Geometry: final body of the model. Coordinates: model frame, mm. Face numbers are marked on the shaded views. A direction names the side the tool comes from. Give positions to 0.01 mm unless a question says otherwise; leave off trailing zeros. Loops run counter-clockwise (first coordinate to the right, second up) from the corner with the lowest first, then second, coordinate; pieces in that order, holes last. Notation, with made-up numbers: (-38.5, 67.5) -> (-2.5, 67.5) arc R23 cw to (-2.5, 82.5) -> close; hole circle Ø1 at (52, 73.25). An arc over 180 degrees is marked (long way). One line per item, written item: value. Start each with the question number.
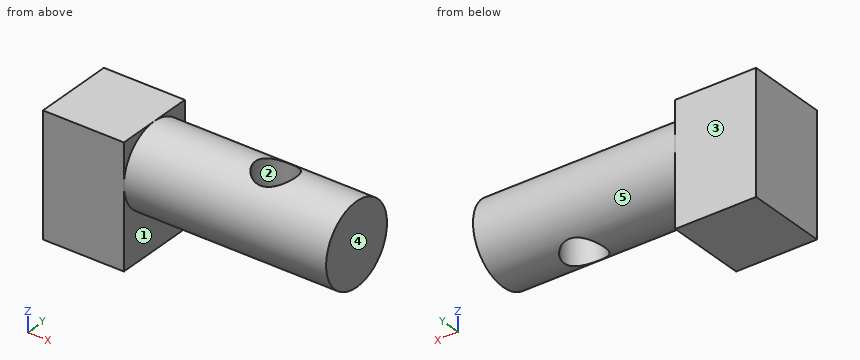
from build123d import *

# Parameters (mm, degrees)
F0_W     = 20
F0_H     = 30
F1_DEPTH = 20
F2_R     = 10
F3_DEPTH = 50
F4_R     = 5
F5_DEPTH = 30.001


with BuildPart() as f1:
    # F0 (on Front) → F1 (new body)
    with BuildSketch(Plane.XZ):
        Rectangle(F0_W, F0_H)
    extrude(amount=F1_DEPTH)

    # F2 (on face) → F3 (join)
    with BuildSketch(Plane.YZ.offset(10)):
        with Locations((-10, 5)):
            Circle(F2_R)
    extrude(amount=F3_DEPTH)

    # F4 (on face) → F5 (cut, through all)
    with BuildSketch(Plane(origin=(0, 0, -15), x_dir=(1, 0, 0), z_dir=(0, 0, -1))):
        with Locations((40, 10)):
            Circle(F4_R)
    extrude(amount=-F5_DEPTH, mode=Mode.SUBTRACT)


solid = f1.part
Item 1: Ray query, line 1 along X through (y, z) = (-10, 1.5); line 2 along Y through (x, z) = (40, 6); line 3 along X through (y, z) = (-14, -5). Return the intervals inside material, ascending. Write a range as [from, to].
Item 2: Mould query, pull axis Y, two halves, no side actions, for the marked faces 1, 2 and 3. Classes: pulls with the +Y half, pulls with the -Y half, needs draft (parallel to the pull), parting line crosses it, or undercut.
Item 3: Access query for the marked faces 4 and 5. Directions: +Z, -Z, +X, -X, +Y, -Y. A direction counts if a zero-diameter tool reaches every point of the face in a straight line with its end or side. Return the directions, or none.
Item 4: Section A-A, the plane z = 3.5. Output: boundary loops of the cut face in (x, y).
Item 5: Section B-B, the plane y = -13.25. Output: boundary loops of the cut face in (x, z), then the cut area to 3 significant figures.
Item 6: Pin query (flat end, axial travel): pin 1 (9 mm diameter, centred on x = 40, y = -10, fed in from +Z); pin 2 (12 mm diameter, centred on x = 47, y = -5.5, fed in from -Z); pin 3 (3 mm diameter, centred on x = 20.5, y = -17, fed in from +Z); pin 4 (1.5 mm diameter, centred on x = 37, z = 5.5, fed in from -Y). Return the tip coordinate at first contact, or that it passes through.
Item 7: Section D-D, the plane x = 27.5. Output: boundary loops of the cut face in (y, z), then the cut area to 3 significant figures.
Item 8: Section C-C, the plane y = -16.25. Output: boundary loops of the cut face in (x, z), then the cut area to 3 significant figures.
Geometry check:
1. line 1: x = [-10, 35], [45, 60]
1. line 2: y = [-19.95, -15], [-5, -0.05]
1. line 3: x = [-10, 10]
2. face 1: needs draft
2. face 2: undercut
2. face 3: pulls with the +Y half
3. face 4: +Z, -Z, +X, +Y, -Y
3. face 5: +X
4. outline: (-10, -20) -> (10, -20) -> (10, -19.89) -> (60, -19.89) -> (60, -0.11) -> (10, -0.11) -> (10, 0) -> (-10, 0) -> close; hole circle Ø10 at (40, -10)
5. outline: (-10, -15) -> (10, -15) -> (10, -4.46) -> (36.2, -4.46) -> (36.2, 14.46) -> (10, 14.46) -> (10, 15) -> (-10, 15) -> close; (43.8, -4.46) -> (60, -4.46) -> (60, 14.46) -> (43.8, 14.46) -> close
5. area: 1,400 mm2
6. pin 1: passes through
6. pin 2: stops at z = -5
6. pin 3: stops at z = 13.35
6. pin 4: stops at y = -20
7. outline: circle Ø20 at (-10, 5)
7. area: 314 mm2
8. outline: (-10, -15) -> (10, -15) -> (10, -2.81) -> (60, -2.81) -> (60, 12.81) -> (10, 12.81) -> (10, 15) -> (-10, 15) -> close
8. area: 1,380 mm2
